```python
from build123d import *

# Parameters (mm, degrees)
EXTRUDE_1_DEPTH     = 20
EXTRUDE_2_DEPTH     = 5
FILLET_1_R          = 10
SKETCH_2_R          = 5
CUT_EXTRUDE_1_DEPTH = 83.006097334
EXTRUDE_5_REACH     = 120.066
EXTRUDE_START       = 35
SKETCH_5_R          = 8
CUT_EXTRUDE_2_DEPTH = 84.066238629


with BuildPart() as part:
    # 草圖1 → 填料-伸長1 (new body)
    with BuildSketch(Plane(origin=(0, 0, 0), x_dir=(0, 0, -1), z_dir=(1, 0, 0))):
        Polygon((5, 0), (0, 0), (0, -10), (35, -10), (35, 0), align=None)
        Polygon((65, 0), (35, 0), (35, -10), (70, -10), (70, 0), align=None)
    extrude(amount=EXTRUDE_1_DEPTH)

    # 草圖1<3> → 填料-伸長2 (add)
    with BuildSketch(Plane(origin=(0, 0, 0), x_dir=(0, 0, -1), z_dir=(1, 0, 0))):
        with BuildLine():
            Line((5, 30), (5, 0))
            Line((5, 0), (35, 0))
            Line((35, 0), (35, 15))
            ThreePointArc((35, 15), (27.928932188, 17.928932188), (25, 25))
            Line((25, 25), (25, 40))
            Line((25, 40), (15, 40))
            ThreePointArc((15, 40), (7.928932188, 37.071067812), (5, 30))
        make_face()
        with BuildLine():
            Line((35, 15), (35, 0))
            Line((35, 0), (65, 0))
            Line((65, 0), (65, 30))
            ThreePointArc((65, 30), (62.071067812, 37.071067812), (55, 40))
            Line((55, 40), (45, 40))
            Line((45, 40), (45, 25))
            ThreePointArc((45, 25), (42.071067812, 17.928932188), (35, 15))
        make_face()
    extrude(amount=EXTRUDE_2_DEPTH)

    # 圓角1
    fillet_1_edges = [part.edges().sort_by_distance(p)[0] for p in [
        (20, -5, 0),
        (20, -5, -70),
    ]]
    fillet(fillet_1_edges, radius=FILLET_1_R)

    # 草圖2 → 除料-伸長1 (cut, through all)
    with BuildSketch(Plane(origin=(5, 0, 0), x_dir=(0, 0, -1), z_dir=(1, 0, 0))):
        with Locations((15, 30)):
            Circle(SKETCH_2_R)
        with Locations((55, 30)):
            Circle(SKETCH_2_R)
    extrude(amount=-CUT_EXTRUDE_1_DEPTH, mode=Mode.SUBTRACT)

    # 填料-伸長5: up to this face of the body (flat: up to its plane)
    extrude_5_end = Plane(part.part.faces().sort_by_distance((5, 32.5, -24.278889745))[0])
    # 草圖3 → 填料-伸長5 (add, up to the picked face)
    with BuildSketch(Plane(origin=(0, 0, 0), x_dir=(0, 0, -1), z_dir=(1, 0, 0)).offset(EXTRUDE_START), mode=Mode.PRIVATE) as extrude_5_sk1:
        with BuildLine():
            Line((17.5, -10), (27, -10))
            ThreePointArc((27, -10), (35, -2), (43, -10))
            Line((43, -10), (52.5, -10))
            ThreePointArc((52.5, -10), (35, 7.5), (17.5, -10))
        make_face()
    extrude_5_tool1 = split(extrude(extrude_5_sk1.sketch, amount=-EXTRUDE_5_REACH, mode=Mode.PRIVATE), bisect_by=extrude_5_end, keep=Keep.BOTH, mode=Mode.PRIVATE)
    add(extrude_5_tool1.solids().sort_by(Axis((35, -1.507575, -35), (-1, 0, 0)))[0])

    # 草圖5 → 除料-伸長2 (cut, through all)
    with BuildSketch(Plane(origin=(20, 0, 0), x_dir=(0, 0, -1), z_dir=(1, 0, 0))):
        with Locations((35, -10)):
            Circle(SKETCH_5_R)
    extrude(amount=-CUT_EXTRUDE_2_DEPTH, mode=Mode.SUBTRACT)


solid = part.part
```
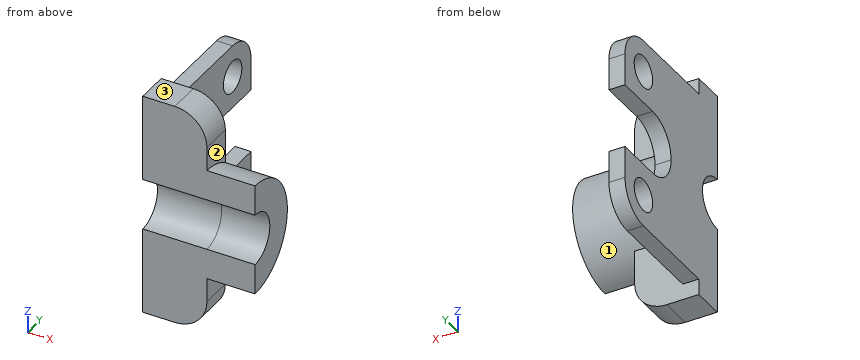
Input: part model. Units: mm. Frame: model coordinates. Face numbers are marked on the shaded views. A direction names the side the tool comes from. Give positions to 0.01 mm unless a question says otherwise; leave off trailing zeros. Write each loop counter-clockwise with the first axis right and the second up, starting at its lowest first coordinate (ties: lowest second). Pieces come first, ordered by that corner, then holes. Notation, with made-up numbers: (4.5, 39.5) - (29.5, 39.5) arc R11 cw to (29.5, 59.5) - close; hole circle Ø3 at (57, 5.25). An arc over 180 degrees is marked (long way). Write item = value, one per line. Start each with the question number.
1. Section query D-D, the plane x = 12.5. Output: boundary loops of the cut face in (y, z).
2. First-contact query: pin 1 Ø13 at (y, z) = (30, -55) entering from +X; pin 2 Ø5.5 at (x, y) = (3, 8.5) entering from -Z; pin 3 Ø5.5 at (x, y) = (2.5, 20.5) entering from +Z; pin 4 Ø9 at (y, z) = (30, -15) entering from +X. Flat tips, straight axial feed; report the tip coordinate or a pass-through.
3. Access query for the marked faces 1, 2 and 3. Directions: +Z, -Z, +X, -X, +Y, -Y. A direction counts if a zero-diameter tool reaches every point of the face in a straight line with its end or side. Return the directions, or none.
4. Section query B-B, the plane x = 3. Output: boundary loops of the cut face in (y, z).
5. Section query A-A, the plane y = 26. Output: boundary loops of the cut face in (x, z), then the cut area to 3 significant figures.
6. Ray query, L1, parallel to Y at x = 3.2, z = -15; L2, parallel to X at y = 21.5, z = -44.5; L3, parallel to Y at x = 16, z = -44. Return the intervals inside material, ascending.
7. Section query C-C, the plane y = -3. Output: boundary loops of the cut face in (x, z).
Check sheet entries:
q1.outline = (-10, -69.68) - (0, -69.68) - (0, -49.36) arc R17.5 ccw to (0, -20.64) - (0, -0.32) - (-10, -0.32) - (-10, -27) arc R8 cw to (-10, -43) - close
q2.pin_1 = 5
q2.pin_2 = -65
q2.pin_3 = -5
q2.pin_4 = through
q3.face_1 = +X, +Y
q3.face_2 = +Z, +X, +Y
q3.face_3 = +Z, +X, -X, +Y, -Y
q4.outline = (-10, -70) - (0, -70) - (0, -65) - (30, -65) arc R10 ccw to (40, -55) - (40, -45) - (25, -45) arc R10 cw to (25, -25) - (40, -25) - (40, -15) arc R10 ccw to (30, -5) - (0, -5) - (0, 0) - (-10, 0) - (-10, -27) arc R8 cw to (-10, -43) - close; hole circle Ø10 at (30, -55); hole circle Ø10 at (30, -15)
q5.outline = (0, -65) - (5, -65) - (5, -58) - (0, -58) - close; (0, -52) - (5, -52) - (5, -45) - (0, -45) - close; (0, -25) - (5, -25) - (5, -18) - (0, -18) - close; (0, -12) - (5, -12) - (5, -5) - (0, -5) - close
q5.area = 140 mm2
q6.L1 = -10 to 25, 35 to 40
q6.L2 = 0 to 5
q6.L3 = -10 to 5.01
q7.outline = (0, -70) - (10, -70) arc R10 ccw to (20, -60) - (20, -51.04) - (35, -51.04) - (35, -38.87) - (0, -38.87) - close; (0, -31.13) - (35, -31.13) - (35, -18.96) - (20, -18.96) - (20, -10) arc R10 ccw to (10, 0) - (0, 0) - close
